Model file for the job. Use its own axes, mm. A direction names the side the tool comes from. Round coordinates to 2 decimals unless told otherwise and drop trailing zeros. Loops run counter-clockwise (first coordinate to the right, second up) from the corner with the lowest first, then second, coordinate; pieces in that order, holes last. Notation, with made-up numbers: (66.5, 47) -> (103.5, 47) arc R23 cw to (103.5, 85) -> close; hole circle Ø5 at (3, 21). An arc over 180 degrees is marked (long way). Use a Markdown table: item, result.
from build123d import *

# Parameters (mm, degrees)
SKETCH_1_W          = 112
SKETCH_1_H          = 52
SKETCH_1_W_2        = 5
SKETCH_1_H_2        = 15
EXTRUDE_1_DEPTH     = 5
MOVE_FACE_1_BY      = 0.1
MOVE_FACE_1_2_BY    = 0.1
MOVE_FACE_1_3_BY    = 0.1
MOVE_FACE_1_4_BY    = 0.1
MOVE_FACE_1_5_BY    = 0.1
MOVE_FACE_1_6_BY    = 0.1
MOVE_FACE_1_7_BY    = 0.1
MOVE_FACE_1_8_BY    = 0.1
MOVE_FACE_1_9_BY    = 0.1
MOVE_FACE_1_10_BY   = 0.1
MOVE_FACE_1_11_BY   = 0.1
MOVE_FACE_1_12_BY   = 0.1
MOVE_FACE_1_13_BY   = 0.1
MOVE_FACE_1_14_BY   = 0.1
MOVE_FACE_1_15_BY   = 0.1
MOVE_FACE_1_16_BY   = 0.1
SKETCH_2_R          = 1.55
CUT_EXTRUDE_1_DEPTH = 5
CUT_EXTRUDE_2_DEPTH = 5
FILLET_1_R          = 2.1
FILLET_2_R          = 10


with BuildPart() as part:
    # 草图1 → 凸台-拉伸1 (new body)
    with BuildSketch(Plane(origin=(0, 0, 0), x_dir=(1, 0, 0), z_dir=(0, 1, 0))):
        Rectangle(SKETCH_1_W, SKETCH_1_H)
        with Locations((42.5, -12.5)):
            Rectangle(SKETCH_1_W_2, SKETCH_1_H_2, mode=Mode.SUBTRACT)
        with Locations((42.5, 12.5)):
            Rectangle(SKETCH_1_W_2, SKETCH_1_H_2, mode=Mode.SUBTRACT)
        with Locations((-42.5, -12.5)):
            Rectangle(SKETCH_1_W_2, SKETCH_1_H_2, mode=Mode.SUBTRACT)
        with Locations((-42.5, 12.5)):
            Rectangle(SKETCH_1_W_2, SKETCH_1_H_2, mode=Mode.SUBTRACT)
    extrude(amount=EXTRUDE_1_DEPTH)

    # Move Face 1: a face moved inward by 0.1
    extrude(part.faces().sort_by_distance((-45, 2.5, -12.5))[0], amount=MOVE_FACE_1_BY, dir=(-1, 0, 0), mode=Mode.SUBTRACT)

    # Move Face 1 2: a face moved inward by 0.1
    extrude(part.faces().sort_by_distance((-42.5, 2.5, -20))[0], amount=MOVE_FACE_1_2_BY, dir=(0, 0, -1), mode=Mode.SUBTRACT)

    # Move Face 1 3: a face moved inward by 0.1
    extrude(part.faces().sort_by_distance((-45, 2.5, 12.5))[0], amount=MOVE_FACE_1_3_BY, dir=(-1, 0, 0), mode=Mode.SUBTRACT)

    # Move Face 1 4: a face moved inward by 0.1
    extrude(part.faces().sort_by_distance((-42.5, 2.5, 5))[0], amount=MOVE_FACE_1_4_BY, dir=(0, 0, -1), mode=Mode.SUBTRACT)

    # Move Face 1 5: a face moved inward by 0.1
    extrude(part.faces().sort_by_distance((-42.5, 2.5, 20))[0], amount=MOVE_FACE_1_5_BY, dir=(0, 0, 1), mode=Mode.SUBTRACT)

    # Move Face 1 6: a face moved inward by 0.1
    extrude(part.faces().sort_by_distance((-40, 2.5, 12.5))[0], amount=MOVE_FACE_1_6_BY, dir=(1, 0, 0), mode=Mode.SUBTRACT)

    # Move Face 1 7: a face moved inward by 0.1
    extrude(part.faces().sort_by_distance((-42.5, 2.5, -5))[0], amount=MOVE_FACE_1_7_BY, dir=(0, 0, 1), mode=Mode.SUBTRACT)

    # Move Face 1 8: a face moved inward by 0.1
    extrude(part.faces().sort_by_distance((-40, 2.5, -12.5))[0], amount=MOVE_FACE_1_8_BY, dir=(1, 0, 0), mode=Mode.SUBTRACT)

    # Move Face 1 9: a face moved inward by 0.1
    extrude(part.faces().sort_by_distance((42.5, 2.5, 20))[0], amount=MOVE_FACE_1_9_BY, dir=(0, 0, 1), mode=Mode.SUBTRACT)

    # Move Face 1 10: a face moved inward by 0.1
    extrude(part.faces().sort_by_distance((40, 2.5, 12.5))[0], amount=MOVE_FACE_1_10_BY, dir=(-1, 0, 0), mode=Mode.SUBTRACT)

    # Move Face 1 11: a face moved inward by 0.1
    extrude(part.faces().sort_by_distance((45, 2.5, 12.5))[0], amount=MOVE_FACE_1_11_BY, dir=(1, 0, 0), mode=Mode.SUBTRACT)

    # Move Face 1 12: a face moved inward by 0.1
    extrude(part.faces().sort_by_distance((42.5, 2.5, 5))[0], amount=MOVE_FACE_1_12_BY, dir=(0, 0, -1), mode=Mode.SUBTRACT)

    # Move Face 1 13: a face moved inward by 0.1
    extrude(part.faces().sort_by_distance((42.5, 2.5, -5))[0], amount=MOVE_FACE_1_13_BY, dir=(0, 0, 1), mode=Mode.SUBTRACT)

    # Move Face 1 14: a face moved inward by 0.1
    extrude(part.faces().sort_by_distance((40, 2.5, -12.5))[0], amount=MOVE_FACE_1_14_BY, dir=(-1, 0, 0), mode=Mode.SUBTRACT)

    # Move Face 1 15: a face moved inward by 0.1
    extrude(part.faces().sort_by_distance((42.5, 2.5, -20))[0], amount=MOVE_FACE_1_15_BY, dir=(0, 0, -1), mode=Mode.SUBTRACT)

    # Move Face 1 16: a face moved inward by 0.1
    extrude(part.faces().sort_by_distance((45, 2.5, -12.5))[0], amount=MOVE_FACE_1_16_BY, dir=(1, 0, 0), mode=Mode.SUBTRACT)

    # 草图2 → 切除-拉伸1 (cut)
    with BuildSketch(Plane(origin=(0, 5, 0), x_dir=(1, 0, 0), z_dir=(0, 1, 0))):
        with Locations((45.1, 18.55)):
            Circle(SKETCH_2_R)
        with Locations((45.1, 6.45)):
            Circle(SKETCH_2_R)
        with Locations((45.1, -6.45)):
            Circle(SKETCH_2_R)
        with Locations((45.1, -18.55)):
            Circle(SKETCH_2_R)
        with Locations((39.9, -18.55)):
            Circle(SKETCH_2_R)
        with Locations((39.9, -6.45)):
            Circle(SKETCH_2_R)
        with Locations((39.9, 6.45)):
            Circle(SKETCH_2_R)
        with Locations((39.9, 18.55)):
            Circle(SKETCH_2_R)
        with Locations((-39.9, 18.55)):
            Circle(SKETCH_2_R)
        with Locations((-39.9, 6.45)):
            Circle(SKETCH_2_R)
        with Locations((-39.9, -6.45)):
            Circle(SKETCH_2_R)
        with Locations((-39.9, -18.55)):
            Circle(SKETCH_2_R)
        with Locations((-45.1, -18.55)):
            Circle(SKETCH_2_R)
        with Locations((-45.1, -6.45)):
            Circle(SKETCH_2_R)
        with Locations((-45.1, 6.45)):
            Circle(SKETCH_2_R)
        with Locations((-45.1, 18.55)):
            Circle(SKETCH_2_R)
    extrude(amount=-CUT_EXTRUDE_1_DEPTH, mode=Mode.SUBTRACT)

    # 草图3 → 切除-拉伸2 (cut)
    with BuildSketch(Plane(origin=(0, 5, 0), x_dir=(1, 0, 0), z_dir=(0, 1, 0))):
        Polygon((2.5, 21), (32.5, 21), (2.5, 6), align=None)
        Polygon((32.5, 16.25), (2.5, 1.25), (32.5, 1.25), align=None)
        Polygon((-2.5, 1.25), (-32.5, 1.25), (-32.5, 16.25), align=None)
        Polygon((-32.5, 21), (-2.5, 6), (-2.5, 21), align=None)
        Polygon((2.5, -1.25), (32.5, -1.25), (32.5, -16.25), align=None)
        Polygon((32.5, -21), (2.5, -6), (2.5, -21), align=None)
        Polygon((-32.5, -1.25), (-32.5, -16.25), (-2.5, -1.25), align=None)
        Polygon((-2.5, -21), (-32.5, -21), (-2.5, -6), align=None)
    extrude(amount=-CUT_EXTRUDE_2_DEPTH, mode=Mode.SUBTRACT)

    # 圆角1
    fillet_1_edges = [part.edges().sort_by_distance(p)[0] for p in [
        (32.5, 2.5, 16.25),
        (2.5, 2.5, 1.25),
        (32.5, 2.5, 1.25),
        (-32.5, 2.5, -21),
        (-2.5, 2.5, -21),
        (-2.5, 2.5, -6),
        (-32.5, 2.5, -16.25),
        (-2.5, 2.5, -1.25),
        (-32.5, 2.5, -1.25),
        (32.5, 2.5, -16.25),
        (32.5, 2.5, -1.25),
        (2.5, 2.5, -1.25),
        (-2.5, 2.5, 6),
        (-2.5, 2.5, 21),
        (-32.5, 2.5, 21),
        (-32.5, 2.5, 1.25),
        (-2.5, 2.5, 1.25),
        (-32.5, 2.5, 16.25),
        (32.5, 2.5, 21),
        (2.5, 2.5, 21),
        (2.5, 2.5, 6),
        (2.5, 2.5, -6),
        (2.5, 2.5, -21),
        (32.5, 2.5, -21),
    ]]
    fillet(fillet_1_edges, radius=FILLET_1_R)

    # 圆角2
    fillet_2_edges = [part.edges().sort_by_distance(p)[0] for p in [
        (-56, 2.5, -26),
        (56, 2.5, -26),
        (56, 2.5, 26),
        (-56, 2.5, 26),
    ]]
    fillet(fillet_2_edges, radius=FILLET_2_R)


solid = part.part
Q1. Flat gauge pin, fed straight in: pin 1 (10 mm diameter, centred on x = 18.5, z = 10.5, fed in from -Y). Where does the tip first touch, or does it go through?
Results list:
| item | result |
|---|---|
| pin 1 | stops at y = 0 |
Q2. Tool access for faces 4 (the face through (-1, 5, 0)), 5 (the face through (-14, 3, -21)): list every direction of +Z, -Z, +X, -X, +Y, -Y with a clear straight run to the whole face (end or side of a thin tool).
Results list:
| item | result |
|---|---|
| face 4 | +Z, -Z, +X, -X, +Y |
| face 5 | +Y, -Y |
Q3. Band-saw the part on C-C, the plane z = 22. Give the cut face in (x, y), plus the area to 3 significant figures.
Results list:
| item | result |
|---|---|
| outline | (-54, 0) -> (54, 0) -> (54, 5) -> (-54, 5) -> close |
| area | 540 mm² |
Q4. Band-saw the part on B-B, the plane x = -7. Give the cut face in (y, z), plus the area to 4 significant figures.
Results list:
| item | result |
|---|---|
| outline | (0, -26) -> (5, -26) -> (5, -21) -> (0, -21) -> close; (0, -8.25) -> (5, -8.25) -> (5, 8.25) -> (0, 8.25) -> close; (0, 21) -> (5, 21) -> (5, 26) -> (0, 26) -> close |
| area | 132.5 mm² |
Q5. Band-saw the part on A-A, the plane x = 15.5. Give the cut face in (y, z).
Results list:
| item | result |
|---|---|
| outline | (0, -26) -> (5, -26) -> (5, -21) -> (0, -21) -> close; (0, -12.5) -> (5, -12.5) -> (5, -7.75) -> (0, -7.75) -> close; (0, -1.25) -> (5, -1.25) -> (5, 1.25) -> (0, 1.25) -> close; (0, 7.75) -> (5, 7.75) -> (5, 12.5) -> (0, 12.5) -> close; (0, 21) -> (5, 21) -> (5, 26) -> (0, 26) -> close |
Q6. Band-saw the part on D-D, the plane y = 0.95. Give the number of separate pieces and of enclosed holes in the cut face, plus the area to 3 significant figures.
Results list:
| item | result |
|---|---|
| separate pieces | 1 |
| enclosed holes | 12 |
| area | 3,690 mm² |
Q7. Pull direction Z, two halves, no side cores. Call faces 1 (the face through (-53.15, 2.54, -22.99)), 2 (the face through (-31.53, 2.46, 14.62)), 3 (the face through (56, 2, 0)): released by +Z, released by -Z, zero draft, split by the parting line, or undercut.
Results list:
| item | result |
|---|---|
| face 1 | released by -Z |
| face 2 | undercut |
| face 3 | zero draft |
Q8. Drill centre lines: L1, parallel to X at y = 2.7, z = -3.5; L2, parallel to Z at x = -9, y = 2; L3, parallel to X at y = 3.6, z = 18. Where is each one in solid material? Low to high. Write a range as from..to.
Results list:
| item | result |
|---|---|
| L1 | x = -56..-32.5, -9.3..9.3, 32.5..56 |
| L2 | z = -26..-21, -9.25..9.25, 21..26 |
| L3 | x = -55.8..-46.55, -38.45..-25.5, -2.5..2.5, 25.5..38.45, 46.55..55.8 |
